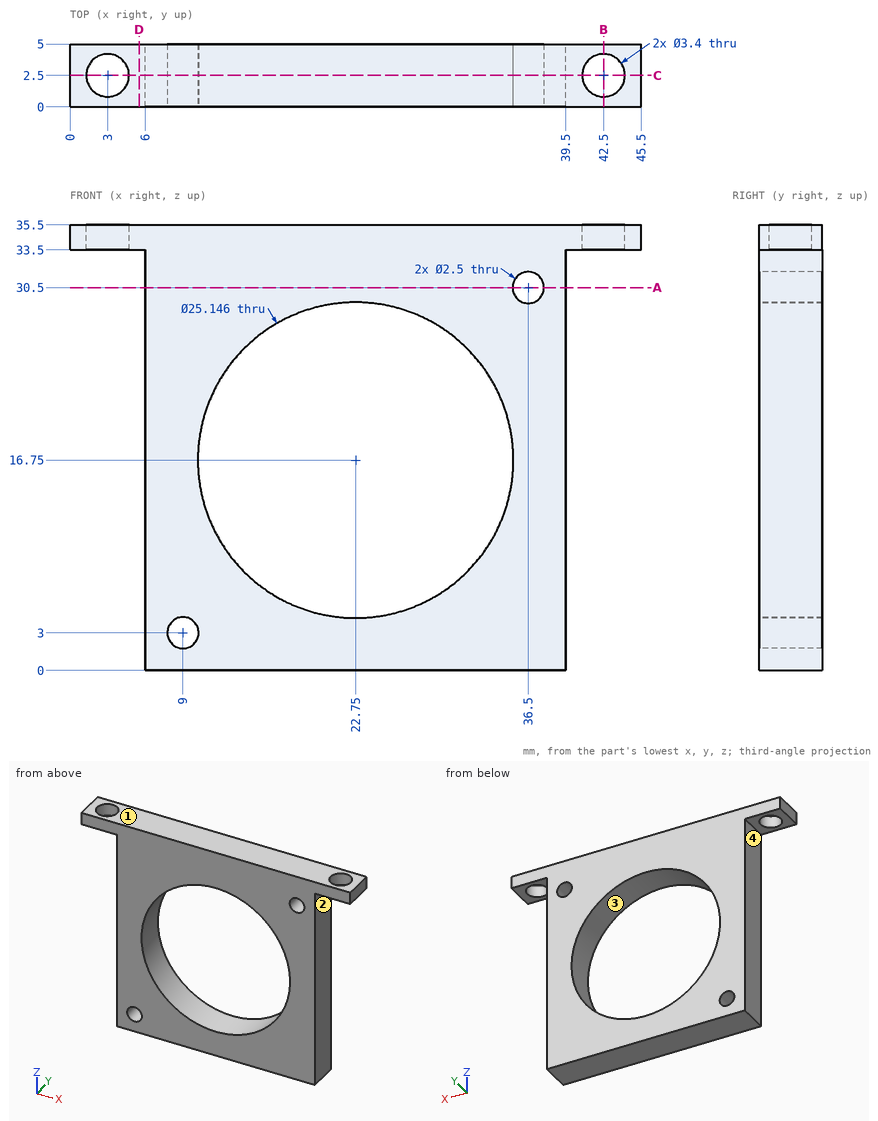
Check sheet for the drawn part. Datum: minimum x, y, z corner. Units: mm. Round coordinates to 2 decimals unless told otherwise and drop trailing zeros. Order: outer loops, then holes, each group sorted by start corner. A loop starts at its lowest first (then second) coordinate and runs counter-clockwise, first axis right, second up.
1. Thickness scan on L1, parallel to Z at x = 22.75, y = 3.55; L2, parallel to Z at x = 42.5, y = 4.85; L3, parallel to Z at x = 18.5, y = 3.9. Record the ranges inside material, lowest first.
Final values:
L1: z = 0 to 4.18, 29.32 to 35.5
L2: z = 33.5 to 35.5
L3: z = 0 to 4.92, 28.58 to 35.5
2. Release check for a two-part mould opening along X. For the marked faces 1, 2, 3 and 4 record: +X half, -X half, draft (parallel to the pull), parting line (faces both ways), or undercut.
Final values:
face 1: draft
face 2: +X half
face 3: undercut
face 4: -X half
3. Section check B-B on x = 42.5. Record the cut outline in (y, z), then the cut area to 3 significant figures.
Final values:
outline: (0, 33.5) - (0.8, 33.5) - (0.8, 35.5) - (0, 35.5) - close; (4.2, 33.5) - (5, 33.5) - (5, 35.5) - (4.2, 35.5) - close
area: 3.20 mm2
4. Section check D-D on x = 5.5. Record the cut outline in (y, z).
Final values:
outline: (0, 33.5) - (5, 33.5) - (5, 35.5) - (0, 35.5) - close
5. Go/stop test with flat-tipped pins: P1, Ø1, axis at y = 3.5, z = 26, coming from the -X side; P2, Ø2.5, axis at x = 4, y = 1.5, coming from the -Z side; P3, Ø1.5, axis at y = 3.5, z = 28.5, coming from the +X side. Record where each tip stops, or that it passes through.
Final values:
P1: stops at x = 6
P2: stops at z = 33.5
P3: stops at x = 39.5
6. Section check A-A on z = 30.5. Record the cut outline in (x, y), then the cut area to 3 significant figures.
Final values:
outline: (6, 0) - (35.25, 0) - (35.25, 5) - (6, 5) - close; (37.75, 0) - (39.5, 0) - (39.5, 5) - (37.75, 5) - close
area: 155 mm2
7. Section check C-C on y = 2.5. Record the cut outline in (x, z), then the cut area to 3 significant figures.
Final values:
outline: (0, 33.5) - (1.3, 33.5) - (1.3, 35.5) - (0, 35.5) - close; (4.7, 33.5) - (6, 33.5) - (6, 0) - (39.5, 0) - (39.5, 33.5) - (40.8, 33.5) - (40.8, 35.5) - (4.7, 35.5) - close; (44.2, 33.5) - (45.5, 33.5) - (45.5, 35.5) - (44.2, 35.5) - close; hole circle Ø2.5 at (9, 3); hole circle Ø25.15 at (22.75, 16.75); hole circle Ø2.5 at (36.5, 30.5)
area: 693 mm2
